Autodesk Inventor part; units mm, degrees
ref_plane "YZ Plane" through (0, 0, 0) normal (1, 0, 0) x (0, 1, 0)
ref_plane "XZ Plane" through (0, 0, 0) normal (0, 1, 0) x (-1, 0, 0)
ref_plane "XY Plane" through (0, 0, 0) normal (0, 0, 1) x (1, 0, 0)
sketch "Sketch1" plane through (0, 0, 0) normal (0, 0, 1) x (1, 0, 0)
  line L0 (-35.3, 51.65) -> (39.3, 51.65)
  line L1 (39.3, 51.65) -> (39.3, -51.65)
  line L2 (39.3, -51.65) -> (-35.3, -51.65)
  line L3 (-35.3, -51.65) -> (-35.3, 51.65)
  line L4 (-35.3, 51.65) -> (39.3, -51.65) construction
  line L5 (39.3, 51.65) -> (-35.3, -51.65) construction
  line L6 (34.3, 26.65) -> (-34.3, 26.65) construction
  line L7 (-34.3, 26.65) -> (-34.3, -26.65) construction
  line L8 (-34.3, -26.65) -> (34.3, -26.65) construction
  line L9 (34.3, -26.65) -> (34.3, 26.65) construction
  line L10 (34.3, 26.65) -> (-34.3, -26.65) construction
  line L11 (-34.3, 26.65) -> (34.3, -26.65) construction
  circle A0 centre (-20.3, 24.05) radius 1.6 construction
  circle A1 centre (-21.6, -24.15) radius 1.6 construction
  circle A2 centre (30.5, 8.85) radius 1.6 construction
  circle A3 centre (30.5, -19.05) radius 1.6 construction
  line L12 (-37.3, 53.65) -> (41.3, 53.65)
  line L13 (41.3, 53.65) -> (41.3, -53.65)
  line L14 (41.3, -53.65) -> (-37.3, -53.65)
  line L15 (-37.3, -53.65) -> (-37.3, 53.65)
  line L16 (-37.3, 53.65) -> (41.3, -53.65) construction
  line L17 (41.3, 53.65) -> (-37.3, -53.65) construction
  line L18 (30.5, 53.65) -> (30.5, -53.65) construction
  arc A4 (27, 53.65) -> (-23, 53.65) centre (2, 53.65) ccw
  arc A5 (-23, -53.65) -> (27, -53.65) centre (2, -53.65) ccw
  circle A6 centre (2, 63.5) radius 4
  circle A7 centre (2, -63.5) radius 4
  line L19 (2, -63.5) -> (2, 63.5) construction
  line L20 (2, 78.65) -> (2, 63.5) construction
  line L21 (2, -63.5) -> (2, -78.65) construction
  point P0 (0, 0)
  dimension "d0" = 53.3
  dimension "d2" = 68.6
  dimension "d3" = 14
  dimension "d4" = 2.5
  dimension "d5" = 50.8
  dimension "d6" = 27.9
  dimension "d7" = 5.1
  dimension "d8" = 3.2
  dimension "d9" = 25
  dimension "d10" = 1
  dimension "d11" = 2
  dimension "d12" = 2
  dimension "d59" = 5
  dimension "d62" = 25
  dimension "d63" = 2
  dimension "d64" = 2
  dimension "d92" = 15.2
  dimension "d94" = 1.3
  dimension "d95" = 50
  dimension "d96" = 8
  dimension "d99" = 127
extrude "Extrusion1" add sketch "Sketch1" against normal blind 2 contours L0 L1 L2 L3 | L12 L13 L14 L15
extrude "Extrusion2" add sketch "Sketch1" along normal blind 50 contours L12 L13 L14 L15
sketch "Sketch2" plane through (0, 0, 0) normal (0, 0, 1) x (1, 0, 0)
  circle A0 centre (-21.6, -24.15) radius 1.6 construction
  circle A1 centre (-20.3, 24.05) radius 4.15
  circle A2 centre (-21.6, -24.15) radius 4.15
  circle A3 centre (30.5, -19.05) radius 4.15
  circle A4 centre (30.5, 8.85) radius 4.15
  circle A5 centre (-20.3, 24.05) radius 2.15
  circle A6 centre (30.5, 8.85) radius 2.15
  circle A7 centre (-21.6, -24.15) radius 2.15
  circle A8 centre (30.5, -19.05) radius 2.15
  point P0 (0, 0)
  dimension "d17" = 8.3
  dimension "d19" = 4.3
extrude "Extrusion3" add sketch "Sketch2" along normal blind 5
sketch "Sketch6" plane through (-37.3, 53.65, -2) normal (0, 1, 0) x (1, 0, 0)
  line L0 (78.6, -52) -> (78.6, 0)
  line L1 (0, 0) -> (0, -52)
  line L2 (0, -42) -> (78.6, -42) construction
  arc A0 (9.2389, -38.11) -> (15.3611, -38.11) centre (12.3, -42) ccw
  line L3 (78.6, -52) -> (0, -52)
  line L4 (12.3, -42) -> (12.3, -38.11) construction
  line L5 (9.2389, -38.11) -> (15.3611, -38.11)
  line L6 (68.6, -46.3) -> (68.6, -39.95)
  line L7 (66.35, -37.7) -> (47.25, -37.7)
  line L8 (45, -39.95) -> (45, -46.3)
  line L9 (45, -46.3) -> (68.6, -46.3)
  line L10 (47.25, -37.7) -> (45, -39.95)
  line L11 (68.6, -39.95) -> (66.35, -37.7)
  line L12 (68.6, -46.3) -> (68.6, -41.3) construction
  line L13 (56.8, -37.7) -> (56.8, -46.3) construction
  point P0 (37.3, -2)
  point P1 (45, -37.7)
  point P2 (68.6, -37.7)
  point P3 (56.8, -42)
  dimension "d46" = 9.9
  dimension "d54" = 12.3
  dimension "d65" = 3.89
  dimension "d122" = 23.6
  dimension "d123" = 8.6
  dimension "d124" = 2.25
  dimension "d125" = 2.25
  dimension "d126" = 2.25
  dimension "d127" = 2.25
  dimension "d128" = 5
  dimension "d129" = 10
  dimension "d130" = 10
extrude "Extrusion6" cut sketch "Sketch6" against normal up to next
sketch "Sketch7" plane through (0, 0, 0) normal (0, 0, 1) x (1, 0, 0)
  circle A0 centre (30.5, -19.05) radius 4.15
  circle A1 centre (30.5, 8.85) radius 4.15
  line L0 (-14.3, -17.05) -> (24.5, -17.05)
  line L1 (24.5, -17.05) -> (24.5, -21.05)
  line L2 (24.5, -21.05) -> (-14.3, -21.05)
  line L3 (-14.3, -21.05) -> (-14.3, -17.05)
  line L4 (-34.3, -26.65) -> (34.3, -26.65) construction
  line L5 (34.3, 26.65) -> (-34.3, 26.65) construction
  line L6 (34.3, -26.65) -> (34.3, 26.65) construction
  line L7 (-34.3, 26.65) -> (-34.3, -26.65) construction
  line L8 (24.5, 16.65) -> (-14.3, 16.65)
  line L9 (-14.3, 16.65) -> (-14.3, 12.65)
  line L10 (-14.3, 12.65) -> (24.5, 12.65)
  line L11 (24.5, 12.65) -> (24.5, 16.65)
  point P0 (0, 0)
  point P1 (24.5, -19.05)
  dimension "d79" = 4
  dimension "d80" = 20
  dimension "d81" = 6
  dimension "d82" = 6
  dimension "d83" = 20
  dimension "d86" = 10
  dimension "d87" = 0
extrude "Extrusion7" add sketch "Sketch7" along normal blind 8 contours L0 L1 L2 L3 | L11 L10 L9 L8
sketch "Sketch4" plane through (-37.3, -53.65, -2) normal (-1, 0, 0) x (0, 0, 1)
  line L0 (11.5, 71.3) -> (23.5, 71.3)
  line L1 (23.5, 71.3) -> (23.5, 58.3)
  line L2 (23.5, 58.3) -> (11.5, 58.3)
  line L3 (11.5, 58.3) -> (11.5, 71.3)
  line L4 (11.5, 71.3) -> (23.5, 58.3) construction
  line L5 (23.5, 71.3) -> (11.5, 58.3) construction
  line L6 (23.5, 30.25) -> (11.5, 30.25)
  line L7 (11.5, 30.25) -> (11.5, 40.25)
  line L8 (11.5, 40.25) -> (23.5, 40.25)
  line L9 (23.5, 40.25) -> (23.5, 30.25)
  line L10 (23.5, 30.25) -> (11.5, 40.25) construction
  line L11 (11.5, 30.25) -> (23.5, 40.25) construction
  line L12 (2, 0) -> (2, 107.3)
  line L13 (7, 73.55) -> (7, 81.85)
  line L14 (10, 36.6) -> (10, 32.6)
  line L15 (0, 107.3) -> (52, 107.3)
  line L16 (0, 0) -> (0, 107.3)
  line L17 (52, 0) -> (0, 0)
  line L18 (52, 107.3) -> (52, 0)
  point P0 (2, 53.65)
  point P1 (2, 80.3)
  point P2 (2, 80.3)
  point P3 (2, 80.3)
  point P4 (2, 27)
  point P5 (2, 27)
  point P6 (2, 27)
  point P7 (17.5, 64.8)
  point P8 (17.5, 35.25)
  point P9 (2, 0)
  dimension "d22" = 13
  dimension "d24" = 12
  dimension "d26" = 9
  dimension "d27" = 12
  dimension "d28" = 10
  dimension "d31" = 3.25
  dimension "d88" = 1.5
  dimension "d90" = 1.5
extrude "Extrusion4" cut sketch "Sketch4" against normal up to surface (2 mm away) contours L0 L1 L2 L3 | L6 L7 L8 L9
extrude "Extrusion8" add sketch "Sketch1" against normal up to surface (2 mm away) contours A4 L12 | L14 A5
sketch "Sketch8" plane through (-37.3, -53.65, 50) normal (0, -1, 0) x (1, 0, 0)
  line L0 (78.6, 0) -> (78.6, -52)
  line L1 (0, 0) -> (78.6, 0)
  line L2 (0, 0) -> (0, -52)
  line L3 (11.5, -5.85) -> (48.5, -5.85)
  line L4 (48.5, -5.85) -> (48.5, -14.15)
  line L5 (48.5, -14.15) -> (11.5, -14.15)
  line L6 (11.5, -14.15) -> (11.5, -5.85)
  line L7 (48.5, -10) -> (52.5, -10) construction
  line L8 (11.5, -10) -> (7.5, -10) construction
  circle A0 centre (7.5, -10) radius 1.5
  circle A1 centre (52.5, -10) radius 1.5
  line L9 (0, -10) -> (7.5, -10) construction
  line L10 (7.5, -10) -> (7.5, 0) construction
  circle A2 centre (68.6, -10) radius 4.05
  line L11 (68.6, -10) -> (68.6, 0) construction
  line L12 (68.6, -10) -> (78.6, -10) construction
  point P0 (37.3, -50)
  dimension "d100" = 8.3
  dimension "d102" = 37
  dimension "d103" = 4
  dimension "d104" = 3
  dimension "d105" = 10
  dimension "d106" = 7.5
  dimension "d107" = 8.1
  dimension "d108" = 10
extrude "Extrusion9" cut sketch "Sketch8" against normal up to next
properties part number "LED pump controller"
The listing builds one solid part. Answer for the finished solid, in the listing's coordinates (mm). A direction names the side the tool comes from. Give positions to 0.01 mm unless a question says otherwise; leave off trailing zeros. Order: outer loops, then holes, each group sorted by start corner. A loop starts at its lowest first (then second) coordinate and runs counter-clockwise, first axis right, second up. Notation, with made-up numbers: (23, 33.25) -> (71, 33.25) arc R27 ccw to (71, 62.25) -> close; hole circle Ø1 at (-15.5, 75). An arc over 180 degrees is marked (long way). One line per item, written item: value.
1) Find section B-B, the plane y = 8.85. Determine the outline of the cut face in (x, z), plus the area to 3 significant figures.
Reported:
outline: (-37.3, -2) -> (41.3, -2) -> (41.3, 50) -> (39.3, 50) -> (39.3, 0) -> (34.65, 0) -> (34.65, 5) -> (32.65, 5) -> (32.65, 0) -> (28.35, 0) -> (28.35, 5) -> (26.35, 5) -> (26.35, 0) -> (-35.3, 0) -> (-35.3, 9.5) -> (-37.3, 9.5) -> close; (-37.3, 21.5) -> (-35.3, 21.5) -> (-35.3, 50) -> (-37.3, 50) -> close
area: 353 mm^2
2) Find section A-A, the plane z = 19. Determine the outline of the cut face in (x, y), plus the area to 3 significant figures.
Reported:
outline: (-37.3, -53.65) -> (41.3, -53.65) -> (41.3, 53.65) -> (-37.3, 53.65) -> (-37.3, 17.65) -> (-35.3, 17.65) -> (-35.3, 51.65) -> (39.3, 51.65) -> (39.3, -51.65) -> (-35.3, -51.65) -> (-35.3, -23.4) -> (-37.3, -23.4) -> close; (-37.3, -13.4) -> (-35.3, -13.4) -> (-35.3, 4.65) -> (-37.3, 4.65) -> close
area: 682 mm^2
3) Find section D-D, the plane y = -10.5. Determine the outline of the cut face in (x, z), plus the area to 3 significant figures.
Reported:
outline: (-37.3, -2) -> (41.3, -2) -> (41.3, 50) -> (39.3, 50) -> (39.3, 0) -> (-35.3, 0) -> (-35.3, 50) -> (-37.3, 50) -> close
area: 357 mm^2
4) Flat-ended cylindrical pins translate along their axes: P1, Ø2, axis at x = -36, z = 18.5, coming from the -Y side; P2, Ø3, axis at x = 32, y = -19.5, coming from the +Z side; P3, Ø5, axis at x = 31.3, z = 40, coming from the -Y side; P4, Ø5, axis at x = 2, y = 63.5, coming from the +Z side (3 decimals). Find the tip coordinate at first contact, or state that the pin passes through.
Reported:
P1: stops at y = -53.65
P2: stops at z = 5
P3: stops at y = 51.65
P4: passes through
5) Determine the mould class of faces 1 (the flat face through (3, -53.65, 24)), 2 (the flat face through (-14.3, -19, 4)), 3 (the flat face through (41.3, 1, 24)) for opening direction Y: pulls with the +Y half, pulls with the -Y half, needs draft (parallel to the pull), parting line crosses it, or undercut.
Reported:
face 1: pulls with the -Y half
face 2: undercut
face 3: needs draft
6) A tool of negligible diameter and unlimited length cuts with its end or side. For faces 4 (the cylindrical face through (1.133, 59.595, -0.986)), 5 (the flat face through (-14.3, 15, 4)), from which of +Z, -Z, +X, -X, +Y, -Y can it reach the whole face along a straight path? Write none if from no direction.
Reported:
face 4: +Z, -Z
face 5: +Z
7) Find the intervals of material crossed by line 1 (X direction, y = 52.7, z = 40); line 2 (X direction, y = -24, z = 2); line 3 (Y direction, x = 2, z = -0.8), in increasing order.
Reported:
line 1: x = -37.3 to -29.95, -20.05 to 7.7, 31.3 to 41.3
line 2: x = -37.3 to -35.3, -25.75 to -23.74, -19.46 to -17.45, 39.3 to 41.3
line 3: y = -78.65 to -67.5, -59.5 to 59.5, 67.5 to 78.65
8) Find section C-C, the plane z = 6.5. Determine the outline of the cut face in (x, y), plus the area to 3 significant figures.
Reported:
outline: (-37.3, -53.65) -> (41.3, -53.65) -> (41.3, 53.65) -> (-37.3, 53.65) -> close; (-14.3, -21.05) -> (24.5, -21.05) -> (24.5, -17.05) -> (-14.3, -17.05) -> close; (-14.3, 12.65) -> (24.5, 12.65) -> (24.5, 16.65) -> (-14.3, 16.65) -> close; hole (-35.3, -51.65) -> (39.3, -51.65) -> (39.3, 51.65) -> (-35.3, 51.65) -> close
area: 1,040 mm^2
